Geometry check sheet. Reference: the model listing, model coordinates, mm. A direction names the side the tool comes from. Round coordinates to 2 decimals unless told otherwise and drop trailing zeros. Write each loop counter-clockwise with the first axis right and the second up, starting at its lowest first coordinate (ties: lowest second). Pieces come first, ordered by that corner, then holes. Notation, with made-up numbers: (32, 61.25) - (79, 61.25) arc R36 ccw to (79, 100.25) - close; hole circle Ø3 at (64.5, 54.5). An arc over 180 degrees is marked (long way). Return JSON: item names as keys, results as strings.
```python
from build123d import *

# Parameters (mm, degrees)
CROQUIS1_W              = 17
CROQUIS1_H              = 27
SALIENTE_EXTRUIR1_DEPTH = 11
CROQUIS2_W              = 17
CROQUIS2_H              = 6
CORTAR_EXTRUIR1_DEPTH   = 6
CROQUIS3_W              = 8
CROQUIS3_H              = 5
CORTAR_EXTRUIR2_DEPTH   = 6
CROQUIS4_W              = 8
CROQUIS4_H              = 5
CORTAR_EXTRUIR3_DEPTH   = 6
CORTAR_EXTRUIR8_DEPTH   = 6
CORTAR_EXTRUIR16_DEPTH  = 2
CORTAR_EXTRUIR17_DEPTH  = 2
CORTAR_EXTRUIR18_DEPTH  = 2
REDONDEO5_START         = -1
REDONDEO5_DEPTH         = 1.04658
REDONDEO5_START_2       = -7.65058
REDONDEO5_2_DEPTH       = 0.804
REDONDEO5_START_3       = -1.866025504
REDONDEO5_3_DEPTH       = 2.366025504
REDONDEO5_START_4       = -8.5
REDONDEO5_4_DEPTH       = 0.84942
REDONDEO5_START_5       = -6.84658
REDONDEO5_5_DEPTH       = 0.712605404
REDONDEO5_START_6       = 3
REDONDEO5_6_DEPTH       = 3
CORTAR_EXTRUIR19_DEPTH  = 17
CORTAR_EXTRUIR20_START  = -10
CORTAR_EXTRUIR20_DEPTH  = 10
REDONDEO6_R             = 1
CORTAR_EXTRUIR21_DEPTH  = 1
CORTAR_EXTRUIR22_DEPTH  = 1
CORTAR_EXTRUIR26_DEPTH  = 1.3
CROQUIS17_W             = 4.267949192
CROQUIS17_H             = 2
CORTAR_EXTRUIR27_DEPTH  = 1.3
CROQUIS19_W             = 4.267949192
CROQUIS19_H             = 1
CORTAR_EXTRUIR28_DEPTH  = 1.3
CROQUIS20_W             = 4.267949192
CROQUIS20_H             = 1
CORTAR_EXTRUIR29_DEPTH  = 1.3


with BuildPart() as part:
    # Croquis1 → Saliente-Extruir1 (new body)
    with BuildSketch(Plane(origin=(0, 0, 0), x_dir=(1, 0, 0), z_dir=(0, 1, 0))):
        Rectangle(CROQUIS1_W, CROQUIS1_H)
    extrude(amount=SALIENTE_EXTRUIR1_DEPTH)

    # Croquis2 → Cortar-Extruir1 (cut)
    with BuildSketch(Plane(origin=(0, 11, 0), x_dir=(1, 0, 0), z_dir=(0, 1, 0))):
        with Locations((0, 10.5)):
            Rectangle(CROQUIS2_W, CROQUIS2_H)
        with Locations((0, -10.5)):
            Rectangle(CROQUIS2_W, CROQUIS2_H)
    extrude(amount=-CORTAR_EXTRUIR1_DEPTH, mode=Mode.SUBTRACT)

    # Croquis3 → Cortar-Extruir2 (cut)
    with BuildSketch(Plane.XY.offset(13.5)):
        with Locations((4.5, 2.5)):
            Rectangle(CROQUIS3_W, CROQUIS3_H)
    extrude(amount=-CORTAR_EXTRUIR2_DEPTH, mode=Mode.SUBTRACT)

    # Croquis4 → Cortar-Extruir3 (cut)
    with BuildSketch(Plane(origin=(0, 0, -13.5), x_dir=(-1, 0, 0), z_dir=(0, 0, -1))):
        with Locations((-4.5, 2.5)):
            Rectangle(CROQUIS4_W, CROQUIS4_H)
    extrude(amount=-CORTAR_EXTRUIR3_DEPTH, mode=Mode.SUBTRACT)

    # Croquis5 → Cortar-Extruir8 (cut)
    with BuildSketch(Plane(origin=(0, 5, 0), x_dir=(1, 0, 0), z_dir=(0, 1, 0))):
        with BuildLine():
            Line((-8.5, 13.5), (-8.5, 9))
            ThreePointArc((-8.5, 9), (-7.181980515, 12.181980515), (-4, 13.5))
            Line((-4, 13.5), (-8.5, 13.5))
        make_face()
        with BuildLine():
            Line((0.5, 13.5), (-4, 13.5))
            ThreePointArc((-4, 13.5), (-0.818019485, 12.181980515), (0.5, 9))
            Line((0.5, 9), (0.5, 13.5))
        make_face()
        with BuildLine():
            ThreePointArc((-4, -13.5), (-7.181980515, -12.181980515), (-8.5, -9))
            Line((-8.5, -9), (-8.5, -13.5))
            Line((-8.5, -13.5), (-4, -13.5))
        make_face()
        with BuildLine():
            ThreePointArc((0.5, -9), (-0.818019485, -12.181980515), (-4, -13.5))
            Line((-4, -13.5), (0.5, -13.5))
            Line((0.5, -13.5), (0.5, -9))
        make_face()
    extrude(amount=-CORTAR_EXTRUIR8_DEPTH, mode=Mode.SUBTRACT)

    # Croquis7 → Cortar-Extruir16 (cut)
    with BuildSketch(Plane(origin=(0, 5, 0), x_dir=(1, 0, 0), z_dir=(0, 1, 0))):
        with BuildLine():
            Line((-8.5, 7.5), (-8.5, 9))
            ThreePointArc((-8.5, 9), (-4, 13.5), (0.5, 9))
            Line((0.5, 9), (0.5, 7.5))
            Line((0.5, 7.5), (-8.5, 7.5))
        make_face()
        with BuildLine():
            Line((-8.5, -9), (-8.5, -7.5))
            Line((-8.5, -7.5), (0.5, -7.5))
            Line((0.5, -7.5), (0.5, -9))
            ThreePointArc((0.5, -9), (-4, -13.5), (-8.5, -9))
        make_face()
    extrude(amount=-CORTAR_EXTRUIR16_DEPTH, mode=Mode.SUBTRACT)

    # Croquis10 → Cortar-Extruir17 (cut)
    with BuildSketch(Plane(origin=(0, 3, 0), x_dir=(1, 0, 0), z_dir=(0, 1, 0))):
        Polygon((-6.133974596, 7.5), (-1.866025404, 7.5), (-1, 9), (-2.5, 11.598076211), (-5.5, 11.598076211), (-7, 9), align=None)
    extrude(amount=-CORTAR_EXTRUIR17_DEPTH, mode=Mode.SUBTRACT)

    # Croquis11 → Cortar-Extruir18 (cut)
    with BuildSketch(Plane(origin=(0, 3, 0), x_dir=(1, 0, 0), z_dir=(0, 1, 0))):
        Polygon((-6.133974596, -7.5), (-1.866025404, -7.5), (-1, -9), (-2.5, -11.598076211), (-5.5, -11.598076211), (-7, -9), align=None)
    extrude(amount=-CORTAR_EXTRUIR18_DEPTH, mode=Mode.SUBTRACT)

    # Redondeo5: read off the stored shape, not the designer's step
    # Redondeo5 outline → Redondeo5 (add)
    with BuildSketch(Plane.YZ.offset(REDONDEO5_START)):
        with BuildLine():
            Line((3, 7.5), (5, 7.5))
            ThreePointArc((5, 7.5), (3.585786438, 8.085786438), (3, 9.5))
            Line((3, 9.5), (3, 7.5))
        make_face()
        with BuildLine():
            ThreePointArc((3, -9.5), (3.585786438, -8.085786438), (5, -7.5))
            Line((5, -7.5), (3, -7.5))
            Line((3, -7.5), (3, -9.5))
        make_face()
    extrude(amount=REDONDEO5_DEPTH)

    # Redondeo5 2 outline → Redondeo5 2 (add)
    with BuildSketch(Plane.YZ.offset(REDONDEO5_START_2)):
        with BuildLine():
            Line((3, 7.5), (5, 7.5))
            ThreePointArc((5, 7.5), (3.585786438, 8.085786438), (3, 9.5))
            Line((3, 9.5), (3, 7.5))
        make_face()
        with BuildLine():
            ThreePointArc((3, -9.5), (3.585786438, -8.085786438), (5, -7.5))
            Line((5, -7.5), (3, -7.5))
            Line((3, -7.5), (3, -9.5))
        make_face()
    extrude(amount=REDONDEO5_2_DEPTH)

    # Redondeo5 3 outline → Redondeo5 3 (add)
    with BuildSketch(Plane.YZ.offset(REDONDEO5_START_3)):
        with BuildLine():
            Line((3, 7.5), (5, 7.5))
            ThreePointArc((5, 7.5), (3.585786438, 8.085786438), (3, 9.5))
            Line((3, 9.5), (3, 7.5))
        make_face()
        with BuildLine():
            ThreePointArc((3, -9.5), (3.585786438, -8.085786438), (5, -7.5))
            Line((5, -7.5), (3, -7.5))
            Line((3, -7.5), (3, -9.5))
        make_face()
    extrude(amount=REDONDEO5_3_DEPTH)

    # Redondeo5 4 outline → Redondeo5 4 (add)
    with BuildSketch(Plane.YZ.offset(REDONDEO5_START_4)):
        with BuildLine():
            Line((3, 7.5), (5, 7.5))
            ThreePointArc((5, 7.5), (3.585786438, 8.085786438), (3, 9.5))
            Line((3, 9.5), (3, 7.5))
        make_face()
        with BuildLine():
            ThreePointArc((3, -9.5), (3.585786438, -8.085786438), (5, -7.5))
            Line((5, -7.5), (3, -7.5))
            Line((3, -7.5), (3, -9.5))
        make_face()
    extrude(amount=REDONDEO5_4_DEPTH)

    # Redondeo5 5 outline → Redondeo5 5 (add)
    with BuildSketch(Plane.YZ.offset(REDONDEO5_START_5)):
        with BuildLine():
            Line((3, 7.5), (5, 7.5))
            ThreePointArc((5, 7.5), (3.585786438, 8.085786438), (3, 9.5))
            Line((3, 9.5), (3, 7.5))
        make_face()
        with BuildLine():
            ThreePointArc((3, -9.5), (3.585786438, -8.085786438), (5, -7.5))
            Line((5, -7.5), (3, -7.5))
            Line((3, -7.5), (3, -9.5))
        make_face()
    extrude(amount=REDONDEO5_5_DEPTH)

    # Redondeo5 6 outline → Redondeo5 6 (cut)
    with BuildSketch(Plane(origin=(0, 0, 0), x_dir=(1, 0, 0), z_dir=(0, 1, 0)).offset(REDONDEO5_START_6)):
        with BuildLine():
            ThreePointArc((0.472135955, 9.5), (0.493028589, 9.250387902), (0.5, 9))
            Line((0.5, 9), (0.5, 9.5))
            Line((0.5, 9.5), (0.472135955, 9.5))
        make_face()
        Polygon((-7, 9), (-6.133974596, 7.5), (-6.133974596, 9.5), (-6.711324865, 9.5), align=None)
        Polygon((-1.866025504, 9.5), (-1.866025504, 7.5), (-1, 9), (-1.288675135, 9.5), align=None)
        with BuildLine():
            Line((-8.5, 9.5), (-8.5, 9))
            ThreePointArc((-8.5, 9), (-8.493028589, 9.250387902), (-8.472135955, 9.5))
            Line((-8.472135955, 9.5), (-8.5, 9.5))
        make_face()
        with BuildLine():
            Line((-8.5, -9), (-8.5, -9.5))
            Line((-8.5, -9.5), (-8.472135955, -9.5))
            ThreePointArc((-8.472135955, -9.5), (-8.493028589, -9.250387902), (-8.5, -9))
        make_face()
        Polygon((-1.866025504, -9.5), (-1.288675135, -9.5), (-1, -9), (-1.866025404, -7.5), align=None)
        Polygon((-6.711324865, -9.5), (-6.133974596, -9.5), (-6.133974596, -7.5), (-7, -9), align=None)
        with BuildLine():
            ThreePointArc((0.5, -9), (0.493028589, -9.250387902), (0.472135955, -9.5))
            Line((0.472135955, -9.5), (0.5, -9.5))
            Line((0.5, -9.5), (0.5, -9))
        make_face()
    extrude(amount=REDONDEO5_6_DEPTH, mode=Mode.SUBTRACT)

    # Croquis12 → Cortar-Extruir19 (cut)
    with BuildSketch(Plane.ZY.offset(8.5)):
        with BuildLine():
            Line((-6.2, 0), (6.2, 0))
            Line((6.2, 0), (6.2, 7.7))
            ThreePointArc((6.2, 7.7), (5.614213562, 9.114213562), (4.2, 9.7))
            Line((4.2, 9.7), (-4.2, 9.7))
            ThreePointArc((-4.2, 9.7), (-5.614213562, 9.114213562), (-6.2, 7.7))
            Line((-6.2, 7.7), (-6.2, 0))
        make_face()
    extrude(amount=-CORTAR_EXTRUIR19_DEPTH, mode=Mode.SUBTRACT)

    # Croquis13 → Cortar-Extruir20 (cut)
    with BuildSketch(Plane(origin=(8.5, 0, 0), x_dir=(0, 0, -1), z_dir=(1, 0, 0)).offset(CORTAR_EXTRUIR20_START)):
        with BuildLine():
            Line((-6.2, 7.7), (-6.2, 9.7))
            Line((-6.2, 9.7), (-4.2, 9.7))
            ThreePointArc((-4.2, 9.7), (-5.614213562, 9.114213562), (-6.2, 7.7))
        make_face()
        with BuildLine():
            Line((6.2, 7.7), (6.2, 9.7))
            Line((6.2, 9.7), (4.2, 9.7))
            ThreePointArc((4.2, 9.7), (5.614213562, 9.114213562), (6.2, 7.7))
        make_face()
    extrude(amount=CORTAR_EXTRUIR20_DEPTH, mode=Mode.SUBTRACT)

    # Redondeo6
    redondeo6_edges = [part.edges().sort_by_distance(p)[0] for p in [
        (0, 11, -7.5),
        (0, 11, 7.5),
    ]]
    fillet(redondeo6_edges, radius=REDONDEO6_R)

    # Croquis14 → Cortar-Extruir21 (cut)
    with BuildSketch(Plane(origin=(0, 1, 0), x_dir=(1, 0, 0), z_dir=(0, 1, 0))):
        with BuildLine():
            Line((-5, 9), (-5, 7.5))
            Line((-5, 7.5), (-3, 7.5))
            Line((-3, 7.5), (-3, 9))
            ThreePointArc((-3, 9), (-4, 10), (-5, 9))
        make_face()
    extrude(amount=-CORTAR_EXTRUIR21_DEPTH, mode=Mode.SUBTRACT)

    # Croquis15 → Cortar-Extruir22 (cut)
    with BuildSketch(Plane(origin=(0, 1, 0), x_dir=(1, 0, 0), z_dir=(0, 1, 0))):
        with BuildLine():
            Line((-5, -9), (-5, -7.5))
            Line((-5, -7.5), (-3, -7.5))
            Line((-3, -7.5), (-3, -9))
            ThreePointArc((-3, -9), (-4, -10), (-5, -9))
        make_face()
    extrude(amount=-CORTAR_EXTRUIR22_DEPTH, mode=Mode.SUBTRACT)

    # Croquis16 → Cortar-Extruir26 (cut)
    with BuildSketch(Plane(origin=(0, 0, -7.5), x_dir=(-1, 0, 0), z_dir=(0, 0, -1))):
        Polygon((1.866025404, 3), (6.133974596, 3), (6.133974596, 1), (5, 1), (3, 1), (1.866025404, 1), align=None)
    extrude(amount=-CORTAR_EXTRUIR26_DEPTH, mode=Mode.SUBTRACT)

    # Croquis17 → Cortar-Extruir27 (cut)
    with BuildSketch(Plane.XY.offset(7.5)):
        with Locations((-4, 2)):
            Rectangle(CROQUIS17_W, CROQUIS17_H)
    extrude(amount=-CORTAR_EXTRUIR27_DEPTH, mode=Mode.SUBTRACT)

    # Croquis19 → Cortar-Extruir28 (cut)
    with BuildSketch(Plane(origin=(0, 0, 6.2), x_dir=(-1, 0, 0), z_dir=(0, 0, -1))):
        with Locations((4, 0.5)):
            Rectangle(CROQUIS19_W, CROQUIS19_H)
    extrude(amount=-CORTAR_EXTRUIR28_DEPTH, mode=Mode.SUBTRACT)

    # Croquis20 → Cortar-Extruir29 (cut)
    with BuildSketch(Plane.XY.offset(-6.2)):
        with Locations((-4, 0.5)):
            Rectangle(CROQUIS20_W, CROQUIS20_H)
    extrude(amount=-CORTAR_EXTRUIR29_DEPTH, mode=Mode.SUBTRACT)


solid = part.part
```
(1) Section check C-C, the plane y = 9. Enter the section's corners in (x, z).
Response values:
{"outline": "(-8.5, -7.5) - (8.5, -7.5) - (8.5, -6.2) - (-1.5, -6.2) - (-1.5, -5.72) - (-8.5, -5.72) - close; (-8.5, 5.72) - (-1.5, 5.72) - (-1.5, 6.2) - (8.5, 6.2) - (8.5, 7.5) - (-8.5, 7.5) - close"}
(2) Section check B-B, the plane x = 3.5. Enter the section's corners in (y, z).
Response values:
{"outline": "(0, -7.5) - (10, -7.5) arc R1 ccw to (11, -6.5) - (11, 6.5) arc R1 ccw to (10, 7.5) - (0, 7.5) - (0, 6.2) - (9.7, 6.2) - (9.7, -6.2) - (0, -6.2) - close"}
(3) Gauge pin test, flat ends, axial feed: pin 1 (2 mm diameter, centred on x = 3, y = 8.5, fed in from -Z); pin 2 (0.8 mm diameter, centred on y = 0.5, z = 8.5, fed in from +X); pin 3 (8 mm diameter, centred on x = 4, z = 0, fed in from -Y). Record the tip position at first contact, or that the pin passes through.
Response values:
{"pin 1": "stops at z = -7.5", "pin 2": "stops at x = 0.5", "pin 3": "stops at y = 9.7"}
(4) Material ranges on line 1 along Z through (x, y) = (1.75, 7); line 2 along Y through (x, z) = (5.25, 0.25); line 3 along Z through (x, y) = (-3, 10), recorded low to high. Write a range as [from, to].
Response values:
{"line 1": "z = [-7.5, -6.2], [6.2, 7.5]", "line 2": "y = [9.7, 11]", "line 3": "z = [-7.5, 7.5]"}
(5) Access from +Z, -Z, +X, -X, +Y, -Y to the whole of each face (thin tool, end or side, straight path). Record for faces 1 (the face through (-4, 3, 12)), 2 (the face through (-3, 1, 10)), 3 (the face through (-6.134, 1, 7)).
Response values:
{"face 1": "+Z, +X, -X, +Y", "face 2": "+Y", "face 3": "-Y"}
(6) Section check A-A, the plane y = 4.25. Enter the section's corners in (x, z), plus the area to 3 significant figures.
Response values:
{"outline": "(-8.5, -7.65) - (-6.22, -7.65) - (-6.13, -7.5) - (-1.87, -7.5) - (-1.78, -7.65) - (0.5, -7.65) - (0.5, -7.5) - (8.5, -7.5) - (8.5, -6.2) - (-8.5, -6.2) - close; (-8.5, 6.2) - (8.5, 6.2) - (8.5, 7.5) - (0.5, 7.5) - (0.5, 7.65) - (-1.78, 7.65) - (-1.87, 7.5) - (-6.13, 7.5) - (-6.22, 7.65) - (-8.5, 7.65) - close", "area": "45.6 mm^2"}
